Source: CAD feature listing. Evaluate the final solid. Frame: model axes, mm. A direction names the side the tool comes from. Coordinates: 2 decimals unless noted, no trailing zeros. Write each loop counter-clockwise with the first axis right and the second up, starting at its lowest first coordinate (ties: lowest second). Pieces come first, ordered by that corner, then holes. Notation, with made-up numbers: (48.25, 29) - (79.25, 29) arc R34 cw to (79.25, 67) - close; hole circle Ø3 at (77, -20). An arc over 180 degrees is marked (long way). One line per item, written item: value.
from build123d import *

# Parameters (mm, degrees)
SKETCH_R     = 18.5
PAD_DEPTH    = 21.5
SKETCH001_R  = 6
PAD001_DEPTH = 6
SKETCH002_R  = 3
PAD002_DEPTH = 15
SKETCH003_R  = 1
POCKET_DEPTH = 5
SKETCH004_R  = 16.5
PAD003_DEPTH = 24.8
SKETCH005_W  = 16
SKETCH005_H  = 7.5
PAD004_DEPTH = 6
SKETCH006_R  = 6.75
PAD005_DEPTH = 8


with BuildPart() as part:
    # Sketch → Pad (new body)
    with BuildSketch(Plane.XY):
        Circle(SKETCH_R)
    extrude(amount=PAD_DEPTH)

    # Sketch001 (on Face2 of Pad) → Pad001 (join)
    with BuildSketch(Plane(origin=(0, 0, 0), x_dir=(1, 0, 0), z_dir=(0, 0, -1))):
        with Locations((7.5, 0)):
            Circle(SKETCH001_R)
    extrude(amount=PAD001_DEPTH)

    # Sketch002 (on Face5 of Pad001) → Pad002 (join)
    with BuildSketch(Plane(origin=(0, 0, -6), x_dir=(1, 0, 0), z_dir=(0, 0, -1))):
        with Locations((7.5, 0)):
            Circle(SKETCH002_R)
    extrude(amount=PAD002_DEPTH)

    # Sketch003 (on Face2 of Pad002) → Pocket (cut)
    with BuildSketch(Plane(origin=(0, 0, 0), x_dir=(1, 0, 0), z_dir=(0, 0, -1))):
        with Locations((0, 15.5)):
            Circle(SKETCH003_R)
        with Locations((13.423394, 7.75)):
            Circle(SKETCH003_R)
        with Locations((13.423394, -7.75)):
            Circle(SKETCH003_R)
        with Locations((0, -15.5)):
            Circle(SKETCH003_R)
        with Locations((-13.423394, -7.75)):
            Circle(SKETCH003_R)
        with Locations((-13.423394, 7.75)):
            Circle(SKETCH003_R)
    extrude(amount=-POCKET_DEPTH, mode=Mode.SUBTRACT)

    # Sketch004 (on Face3 of Pocket) → Pad003 (join)
    with BuildSketch(Plane.XY.offset(21.5)):
        Circle(SKETCH004_R)
    extrude(amount=PAD003_DEPTH)

    # Sketch005 (on Face19 of Pad003) → Pad004 (join)
    with BuildSketch(Plane.XY.offset(46.3)):
        with Locations((0, 11.75)):
            Rectangle(SKETCH005_W, SKETCH005_H)
    extrude(amount=PAD004_DEPTH)

    # Sketch006 (on Face19 of Pad004) → Pad005 (join)
    with BuildSketch(Plane.XY.offset(46.3)):
        Circle(SKETCH006_R)
    extrude(amount=PAD005_DEPTH)


solid = part.part
1) Draft query along Y for faces 5 (the flat face through (8, 12, 49)), 6 (the cylindrical face through (15.24, -6.32, 33.73)), 7 (the cylindrical face through (-0.217, 16.476, 2.465)). Return one class per face: released by +Y, released by -Y, zero draft, split by the parting line, or undercut.
Values found:
face 5: zero draft
face 6: split by the parting line
face 7: undercut
2) Section query B-B on x = 0. Output: boundary loops of the cut face in (y, z), then the cut area to 3 significant figures.
Values found:
outline: (-18.5, 0) - (-16.5, 0) - (-16.5, 5) - (-14.5, 5) - (-14.5, 0) - (14.5, 0) - (14.5, 5) - (16.5, 5) - (16.5, 0) - (18.5, 0) - (18.5, 21.5) - (16.5, 21.5) - (16.5, 46.3) - (15.5, 46.3) - (15.5, 52.3) - (8, 52.3) - (8, 46.3) - (6.75, 46.3) - (6.75, 54.3) - (-6.75, 54.3) - (-6.75, 46.3) - (-16.5, 46.3) - (-16.5, 21.5) - (-18.5, 21.5) - close
area: 1,750 mm2
3) Material intervals for line 1 (Y direction, x = 0, z = 2); line 2 (X direction, y = 7.75, z = 2.35); line 3 (X direction, y = -7, z = 3), sorted ascending.
Values found:
line 1: -18.5 to -16.5, -14.5 to 14.5, 16.5 to 18.5
line 2: -16.8 to -14.42, -12.42 to 12.42, 14.42 to 16.8
line 3: -17.12 to -14.08, -12.76 to 12.76, 14.08 to 17.12
4) Section query D-D on y = -15.5. Output: boundary loops of the cut face in (x, z), then the cut area to 3 significant figures.
Values found:
outline: (-10.1, 0) - (-1, 0) - (-1, 5) - (1, 5) - (1, 0) - (10.1, 0) - (10.1, 21.5) - (5.66, 21.5) - (5.66, 46.3) - (-5.66, 46.3) - (-5.66, 21.5) - (-10.1, 21.5) - close
area: 705 mm2
5) Section query A-A on y = 0. Output: boundary loops of the cut face in (x, z).
Values found:
outline: (-18.5, 0) - (1.5, 0) - (1.5, -6) - (4.5, -6) - (4.5, -21) - (10.5, -21) - (10.5, -6) - (13.5, -6) - (13.5, 0) - (18.5, 0) - (18.5, 21.5) - (16.5, 21.5) - (16.5, 46.3) - (6.75, 46.3) - (6.75, 54.3) - (-6.75, 54.3) - (-6.75, 46.3) - (-16.5, 46.3) - (-16.5, 21.5) - (-18.5, 21.5) - close
6) Contact query for flat-ended pins moving along their axis: P1, Ø5, axis at y = 0, z = -8, coming from the +X side; P2, Ø2, axis at x = 3.5, y = 10.5, coming from the +Z side; P3, Ø1.8, axis at x = 0, y = -15.5, coming from the -Z side. Output: stop coordinate, or through.
Values found:
P1: x = 13.5
P2: z = 52.3
P3: z = 5
7) Section query C-C on z = 12.5. Output: boundary loops of the cut face in (x, y), then the cut area to 3 significant figures.
Values found:
outline: circle Ø37 at (0, 0)
area: 1,080 mm2
8) Reachability of faces 1 (the flat face through (0, 8, 49)), 2 (the flat face through (-8, 12, 49)), 3 (the flat face through (0, 12, 52.3)), 4 (the flat face through (0, -16, 5)) from +Z, -Z, +X, -X, +Y, -Y: full face, straight path, thin tool, end or side. Return the list, or none.
Values found:
face 1: +Z, +X, -X
face 2: +Z, -X, +Y, -Y
face 3: +Z, +X, -X, +Y
face 4: -Z
